Print and shaded views of the part. All mm, measured from the part's lowest x, y and z. A direction names the side the tool comes from. Round coordinates to 2 decimals unless told otherwise and drop trailing zeros. Order: outer loops, then holes, each group sorted by start corner. A loop starts at its lowest first (then second) coordinate and runs counter-clockwise, first axis right, second up. Notation, with made-up numbers: (-39.75, 73) - (-22.75, 73) arc R19 ccw to (-22.75, 90) - close; hole circle Ø9 at (57, 30.5). An arc over 180 degrees is marked (long way). Return JSON: item names as keys, results as strings. Group by question number.
Item 1: Drop flat-ended pins along their axis: pin 1 (1.5 mm diameter, centred on x = 3.5, z = 6.5, fed in from +Y); pin 2 (4.5 mm diameter, centred on y = 4, z = 4, fed in from +X); pin 3 (1 mm diameter, centred on x = 8.5, z = 6, fed in from -Y). Give the stop position or say it passes through.
Item 2: Saw through at D-D on x = 2.5. List the corners of the cut face in (y, z).
Item 3: Tool access for the marked faces 1, 2 and 3: list every direction of +Z, -Z, +X, -X, +Y, -Y with a clear straight run to the whole face (end or side of a thin tool).
Item 4: Saw through at A-A on x = 10. List the corners of the cut face in (y, z).
Item 5: Two-plate mould, pull along Y, no slides. Class the marked faces 4, 5 and 6: released by +Y, released by -Y, zero draft, split by the parting line, or undercut.
Item 6: Probe probe 1 along X at (y, z) = (2, 7.25); probe 2 along X at (y, z) = (4, 7.2); probe 3 along Z at (x, y) = (12, 4). List the from-to ranges inside material, lowest first.
Item 7: Saw through at C-C on x = 12.5. List the corners of the cut face in (y, z).
Item 8: Saw through at B-B on y = 4. State how many separate pieces and enclosed holes the cut face has, and give its area (3 significant figures).
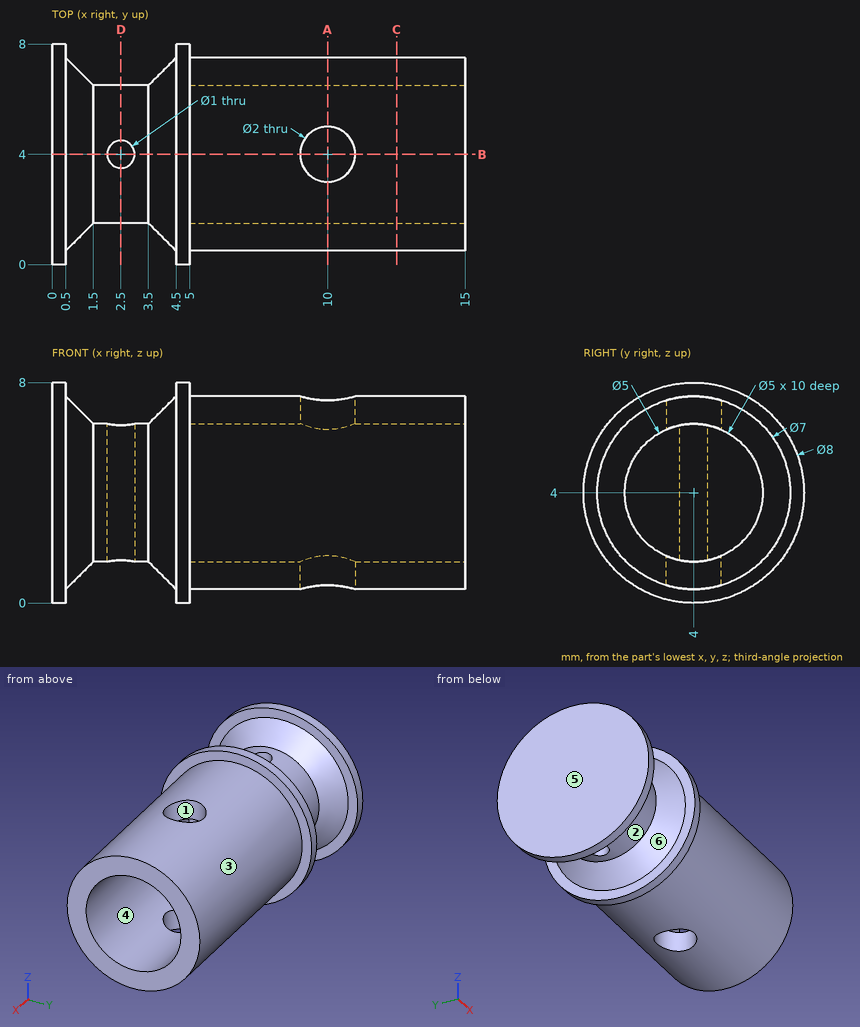
Filled in:
{
 "1": {"pin 1": "stops at y = 6.33", "pin 2": "stops at x = 5", "pin 3": "stops at y = 0.84"},
 "2": {"outline": "(3.5, 1.55) - (3.5, 6.45) arc R2.5 ccw to start; (4.5, 1.55) arc R2.5 ccw to (4.5, 6.45) - close"},
 "3": {"face 1": "+Z, -Z", "face 2": "none", "face 3": "+X"},
 "4": {"outline": "(3, 0.65) - (3, 1.71) arc R2.5 cw to (3, 6.29) - (3, 7.35) arc R3.5 ccw to start; (5, 0.65) arc R3.5 ccw to (5, 7.35) - (5, 6.29) arc R2.5 cw to (5, 1.71) - close"},
 "5": {"face 4": "undercut", "face 5": "zero draft", "face 6": "split by the parting line"},
 "6": {"probe 1": "x = 0 to 0.5, 4.5 to 5", "probe 2": "x = 0 to 0.8, 4.2 to 9, 11 to 15", "probe 3": "z = 0.5 to 1.5, 6.5 to 7.5"},
 "7": {"outline": "circle Ø7 at (4, 4); hole circle Ø5 at (4, 4)"},
 "8": {"separate pieces": "4", "enclosed holes": "0", "area": "41.0 mm^2"}
}
